```python
from build123d import *

# Parameters (mm, degrees)
BOSS_EXTRUDE1_DEPTH = 2.65684
SKETCH2_R           = 76.2
CUT_EXTRUDE1_DEPTH  = 3.65684
SKETCH3_R           = 6.35
CUT_EXTRUDE2_DEPTH  = 3.65684


with BuildPart() as part:
    # Sketch1 → Boss-Extrude1 (new body)
    with BuildSketch(Plane(origin=(0, 0, 0), x_dir=(1, 0, 0), z_dir=(0, 1, 0))):
        Polygon((0, 450.85), (0, 0), (546.1, 0), (546.1, 25.4), align=None)
    extrude(amount=BOSS_EXTRUDE1_DEPTH)

    # Sketch2 → Cut-Extrude1 (cut, through all)
    with BuildSketch(Plane.XZ):
        with Locations((254, -114.3)):
            Circle(SKETCH2_R)
    extrude(amount=-CUT_EXTRUDE1_DEPTH, mode=Mode.SUBTRACT)

    # Sketch3 → Cut-Extrude2 (cut, through all)
    with BuildSketch(Plane.XZ):
        with Locations((344.060644326, -83.289633288)):
            Circle(SKETCH3_R)
        with Locations((235.82544319, -207.799989223)):
            Circle(SKETCH3_R)
        with Locations((182.113912484, -51.810377489)):
            Circle(SKETCH3_R)
    extrude(amount=-CUT_EXTRUDE2_DEPTH, mode=Mode.SUBTRACT)


solid = part.part
```
Can you work these out from the model? Positions are in its coordinate system, mm. Coordinates: 2 decimals unless noted, no trailing zeros. Order: outer loops, then holes, each group sorted by start corner. A loop starts at its lowest first (then second) coordinate and runs counter-clockwise, first axis right, second up. Notation, with made-up numbers: (87.5, 45) -> (109.5, 45) arc R12 cw to (109.5, 53) -> close; hole circle Ø7 at (60, -26). An arc over 180 degrees is marked (long way). Write each question's results on one line, items separated by ' | '.
Item 1: I want a section at C-C, the plane y = 2.1. Write out the boundary of the cut face in (x, z).
Results are:
outline: (0, -450.85) -> (546.1, -25.4) -> (546.1, 0) -> (0, 0) -> close; hole circle Ø12.7 at (182.11, -51.81); hole circle Ø152.4 at (254, -114.3); hole circle Ø12.7 at (235.83, -207.8); hole circle Ø12.7 at (344.06, -83.29)
Item 2: I'm going to push flat-ended pins straight in: pin 1 Ø3 at (x, z) = (128, -353.5) entering from -Y; pin 2 Ø1.5 at (y, z) = (1.5, -309.5) entering from +X. Where does each tip first touch, or does it pass through?
Results are:
pin 1: through | pin 2: x = 182.4
Item 3: If I drill on line 1 along Z through (x, y) = (226.5, 1.6); line 2 along Z through (x, y) = (219.5, 0.75); line 3 along X through (y, z) = (1.65, -182.5), over which ranges is the centre line in solid material (lowest first)?
Results are:
line 1: -274.39 to -185.36, -43.24 to 0 | line 2: -279.84 to -182.24, -46.36 to 0 | line 3: 0 to 220.01, 287.99 to 344.45
Item 4: I want a section at B-B, the plane z = -114.3. Write out the boundary of the cut face in (x, y).
Results are:
outline: (0, 0) -> (177.8, 0) -> (177.8, 2.66) -> (0, 2.66) -> close; (330.2, 0) -> (431.99, 0) -> (431.99, 2.66) -> (330.2, 2.66) -> close
Item 5: I want a section at A-A, the plane x = 277. Write out the boundary of the cut face in (y, z).
Results are:
outline: (0, -235.05) -> (2.66, -235.05) -> (2.66, -186.95) -> (0, -186.95) -> close; (0, -41.65) -> (2.66, -41.65) -> (2.66, 0) -> (0, 0) -> close
Item 6: If we mould it in two halves opening along X, with no side actions, what happens to faces 1 (the face through (209, 0, -178)), 2 (the face through (197.84, 1.31, -62.8)), 3 (the face through (339.02, 1.31, -87.15)), 4 (the face through (276.87, 1.31, -235.15))? For each: +X half, -X half, draft (parallel to the pull), parting line (faces both ways), or undercut.
Results are:
face 1: draft | face 2: undercut | face 3: undercut | face 4: +X half
Item 7: I want a section at D-D, the plane x = 486. Write out the boundary of the cut face in (y, z).
Results are:
outline: (0, -72.22) -> (2.66, -72.22) -> (2.66, 0) -> (0, 0) -> close
